```python
from build123d import *

# Parameters (mm, degrees)
REDONDEO1_R            = 2
TALADRO_ROSCADO_M61_D  = 5
TALADRO_ROSCADO_M141_D = 12
MATRIZC1_COUNT         = 6


with BuildPart() as part:
    # Croquis1 → Revolución1 (revolve)
    with BuildSketch(Plane.XY, mode=Mode.PRIVATE) as revoluci_n1_sk:
        Polygon((2, 0), (2, 15), (35, 15), (35, 5), (15, 5), (15, 0), align=None)
    revolve(revoluci_n1_sk.sketch.rotate(Axis((0, 0, 0), (0, 1, 0)), 90), axis=Axis((0, 0, 0), (0, 1, 0)))

    # Redondeo1
    redondeo1_edges = [part.edges().sort_by_distance(p)[0] for p in [
        (0, 5, 15),
    ]]
    fillet(redondeo1_edges, radius=REDONDEO1_R)

    # Taladro roscado M61 (through all)
    with Locations(Plane(origin=(0, 15, 0), x_dir=(1, 0, 0), z_dir=(0, 1, 0))):
        with Locations((29, 0)):
            taladro_roscado_m61 = Hole(TALADRO_ROSCADO_M61_D / 2)

    # Taladro roscado M141 (through all)
    with Locations(Plane(origin=(0, 15, 0), x_dir=(1, 0, 0), z_dir=(0, 1, 0))):
        with Locations((0, 0)):
            Hole(TALADRO_ROSCADO_M141_D / 2)

    # MatrizC1: Taladro roscado M61 ×6 about axis
    matrizc1_axis = Axis((0, 0, 0), (0, 1, 0))
    for i in range(1, MATRIZC1_COUNT):
        add(taladro_roscado_m61.rotate(matrizc1_axis, i * 360 / MATRIZC1_COUNT), mode=Mode.SUBTRACT)


solid = part.part
```
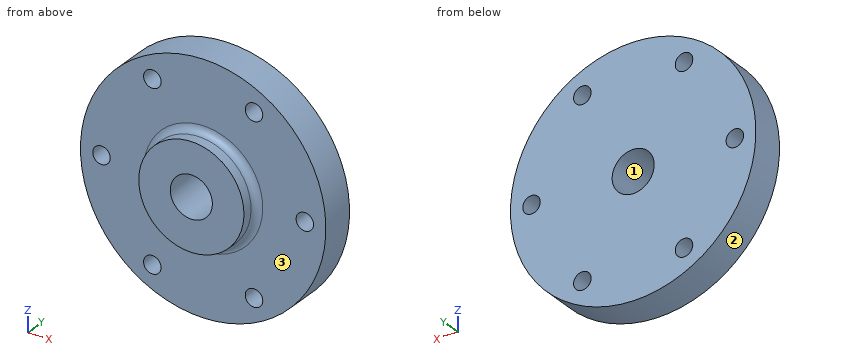
Here's how the part is built. I have some questions about the finished solid (model axes, mm). Face numbers are marked on the shaded views. Coordinates: 2 decimals unless noted, no trailing zeros. Write each loop counter-clockwise with the first axis right and the second up, starting at its lowest first coordinate (ties: lowest second). Pieces come first, ordered by that corner, then holes. Notation, with made-up numbers: M 28,9.5 L 50,9.5 A6 cw 50,19.5 Z; hole C 61,4.25 d1. An arc over 180 degrees is marked long. Answer as CSV lines item,"result". Start each with the question number.
Q1. If we mould it in two halves opening along Z, with no side actions, what happens to the marked faces 1, 2 and 3? For each: pulls with the +Z half, pulls with the -Z half, needs draft (parallel to the pull), parting line crosses it, or undercut.
Q2. I need wall thicknesses on probe 1 along Z at (x, y) = (-14.5, 7); probe 2 along X at (y, z) = (10.75, 25.5); probe 3 along Y at (x, z) = (-17, -2.5). Which ranges of each line are inside material? Lowest first, please. Write a range as [from, to].
Q3. Suppose I cut it at B-B, the plane z = 0. List the corners of the cut face in (x, y) for me, then the cut area to 3 significant figures.
Q4. Will these pins go through, and if not, where does the flat tip stop? pin 1 Ø6 at (x, y) = (-6, 8) entering from +Z; pin 2 Ø2 at (y, z) = (5, -7) entering from -X; pin 3 Ø8 at (x, y) = (-28, 2) entering from +Z.
Q5. Suppose I cut it at C-C, the plane y = 12.75. List the corners of the cut face in (x, z) for me.
Q6. Suppose I cut it at D-D, the plane z = -24. List the corners of the cut face in (x, y) for me, then the cut area to 3 significant figures.
Q7. Suppose I cut it at A-A, the plane x = 0. List the corners of the cut face in (y, z) for me, then the cut area to 3 significant figures.
Entries:
1,face 1,"undercut"
1,face 2,"parting line crosses it"
1,face 3,"needs draft"
2,probe 1,"z = [-31.86, -27.61], [-22.61, 22.61], [27.61, 31.86]"
2,probe 2,"x = [-23.97, -16.97], [-12.03, 12.03], [16.97, 23.97]"
2,probe 3,"y = [5, 15]"
3,outline,"M -35,5 L -31.5,5 L -31.5,15 L -35,15 Z; M -26.5,5 L -17,5 A2 cw -15,3 L -15,0 L -6,0 L -6,15 L -26.5,15 Z; M 6,0 L 15,0 L 15,3 A2 cw 17,5 L 26.5,5 L 26.5,15 L 6,15 Z; M 31.5,5 L 35,5 L 35,15 L 31.5,15 Z"
3,area,"572 mm²"
4,pin 1,"stops at z = 34.87"
4,pin 2,"stops at x = -34.48"
4,pin 3,"stops at z = 24.13"
5,outline,"C 0,0 d70; hole C -29,0 d5; hole C -14.5,-25.11 d5; hole C -14.5,25.11 d5; hole C 0,0 d12; hole C 14.5,-25.11 d5; hole C 14.5,25.11 d5; hole C 29,0 d5"
6,outline,"M -25.48,5 L -16.74,5 L -16.74,15 L -25.48,15 Z; M -12.26,5 L 12.26,5 L 12.26,15 L -12.26,15 Z; M 16.74,5 L 25.48,5 L 25.48,15 L 16.74,15 Z"
6,area,"420 mm²"
7,outline,"M 0,-15 L 3,-15 A2 cw 5,-17 L 5,-35 L 15,-35 L 15,-6 L 0,-6 Z; M 0,6 L 15,6 L 15,35 L 5,35 L 5,17 A2 cw 3,15 L 0,15 Z"
7,area,"672 mm²"
